Here's the drawing with two shaded views (mm, measured from the low corner). I have some questions. Give positions to 0.01 mm unless a question says otherwise; leave off trailing zeros. Loops run counter-clockwise (first coordinate to the right, second up) from the corner with the lowest first, then second, coordinate; pieces in that order, holes last. Notation, with made-up numbers: (83.5, -36) - (139.5, -36) arc R17 ccw to (139.5, -22) - close; hole circle Ø1 at (16, -24). An arc over 180 degrees is marked (long way). Write each question's results on one line, items separated by ' | '. Start each with the question number.
1) I want a section at C-C, the plane z = 24. Write out the boundary of the cut face in (x, y) (3 decimals).
2) If I drill on probe 1 along Z at (x, y) = (22, 0.95) (3 decimals); probe 2 along Z at (x, y) = (20, 1.4) (3 decimals); probe 3 along X at (y, z) = (1.65, 32) (3 decimals), over which ranges is the centre line in solid material (lowest first)? Write a range as [from, to].
3) I want a section at A-A, the plane x = 23. Write out the boundary of the cut face in (y, z) (3 decimals).
4) I'm going to push flat-ended pins straight in: pin 1 (1.5 mm diameter, centred on y = 1.5, z = 20.5, fed in from -X) (3 decimals); pin 2 (0.8 mm diameter, centred on x = 1, y = 1.5, fed in from -Z) (3 decimals); pin 3 (1.3 mm diameter, centred on y = 1, z = 1.5, fed in from -X). Where does each tip first touch, or does it pass through?
5) I want a section at B-B, the plane y = 1.75. Write out the boundary of the cut face in (x, z) (3 decimals).
6) I want a section at D-D, the plane x = 18. Write out the boundary of the cut face in (y, z) (3 decimals), and give its area (3 significant figures).
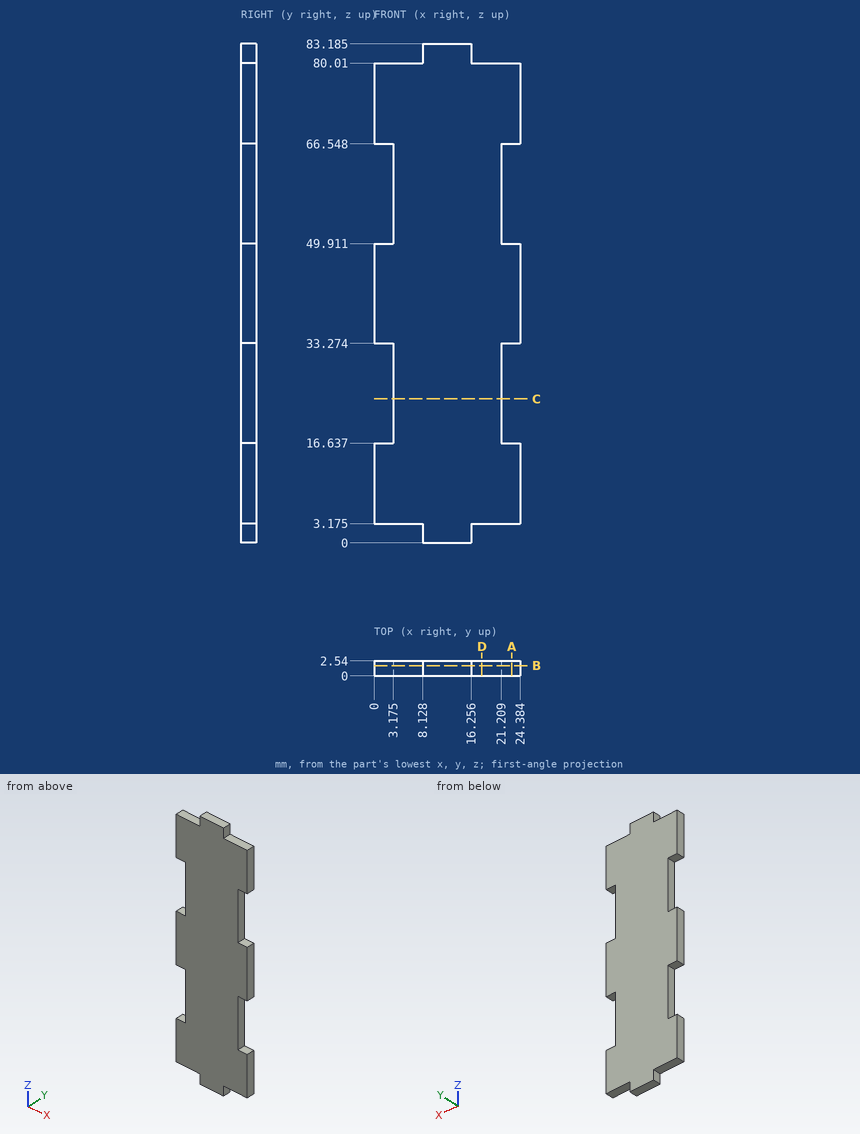
Answers:
1) outline: (3.175, 0) - (21.209, 0) - (21.209, 2.54) - (3.175, 2.54) - close
2) probe 1: z = [3.175, 16.637], [33.274, 49.911], [66.548, 80.01] | probe 2: z = [3.175, 80.01] | probe 3: x = [3.175, 21.209]
3) outline: (0, 3.175) - (2.54, 3.175) - (2.54, 16.637) - (0, 16.637) - close; (0, 33.274) - (2.54, 33.274) - (2.54, 49.911) - (0, 49.911) - close; (0, 66.548) - (2.54, 66.548) - (2.54, 80.01) - (0, 80.01) - close
4) pin 1: stops at x = 3.175 | pin 2: stops at z = 3.175 | pin 3: stops at x = 8.13
5) outline: (0, 3.175) - (8.128, 3.175) - (8.128, 0) - (16.256, 0) - (16.256, 3.175) - (24.384, 3.175) - (24.384, 16.637) - (21.209, 16.637) - (21.209, 33.274) - (24.384, 33.274) - (24.384, 49.911) - (21.209, 49.911) - (21.209, 66.548) - (24.384, 66.548) - (24.384, 80.01) - (16.256, 80.01) - (16.256, 83.185) - (8.128, 83.185) - (8.128, 80.01) - (0, 80.01) - (0, 66.548) - (3.175, 66.548) - (3.175, 49.911) - (0, 49.911) - (0, 33.274) - (3.175, 33.274) - (3.175, 16.637) - (0, 16.637) - close
6) outline: (0, 3.175) - (2.54, 3.175) - (2.54, 80.01) - (0, 80.01) - close | area: 195 mm2
